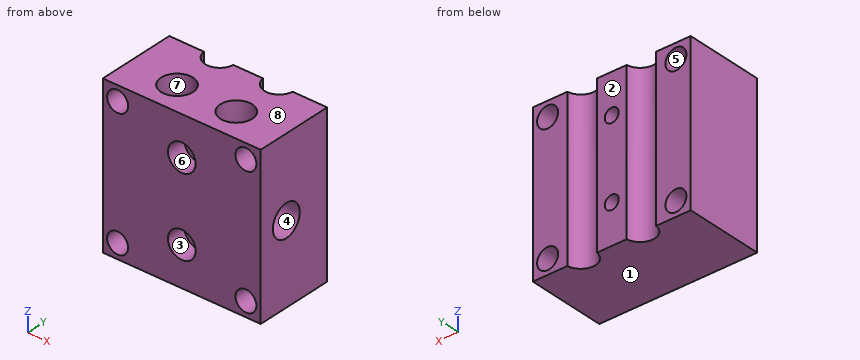
from build123d import *

# Parameters (mm, degrees)
SKETCH1_W                         = 50.8
SKETCH1_H                         = 50.8
BOSS_EXTRUDE1_DEPTH               = 25.4
SKETCH2_R                         = 4.7625
CUT_EXTRUDE1_DEPTH                = 63.217039467
F_1_4_CLEARANCE_HOLE1_D           = 6.7564
F_8_CLEARANCE_HOLE1_D             = 4.4958
SKETCH9_R                         = 4.445
CUT_EXTRUDE3_DEPTH                = 6.35
F_1_8_NPT_TAPPED_HOLE1_AT_2_COUNT = 2
F_1_8_NPT_TAPPED_HOLE1_AT_2_PITCH = 19.05


with BuildPart() as part:
    # Sketch1 → Boss-Extrude1 (new body)
    with BuildSketch(Plane(origin=(0, 0, 0), x_dir=(1, 0, 0), z_dir=(0, 1, 0))):
        Rectangle(SKETCH1_W, SKETCH1_H)
    extrude(amount=BOSS_EXTRUDE1_DEPTH)

    # Sketch2 → Cut-Extrude1 (cut, through all)
    with BuildSketch(Plane.XY.offset(25.4)):
        with Locations((-9.525, 25.908)):
            Circle(SKETCH2_R)
        with Locations((9.525, 25.908)):
            Circle(SKETCH2_R)
    extrude(amount=-CUT_EXTRUDE1_DEPTH, mode=Mode.SUBTRACT)

    # 1/4 Clearance Hole1 (through all)
    with Locations(Plane(origin=(0, 25.4, 0), x_dir=(1, 0, 0), z_dir=(0, 1, 0))):
        with Locations((-20.6375, 20.6375), (-20.6375, -20.6375), (20.6375, -20.6375), (20.6375, 20.6375)):
            Hole(F_1_4_CLEARANCE_HOLE1_D / 2)

    # #8 Clearance Hole1 (through all)
    with Locations(Plane(origin=(0, 25.4, 0), x_dir=(1, 0, 0), z_dir=(0, 1, 0))):
        with Locations((0, 12.7), (0, -12.7)):
            Hole(F_8_CLEARANCE_HOLE1_D / 2)

    # Sketch9 → Cut-Extrude3 (cut)
    with BuildSketch(Plane.XZ):
        with Locations(Location((0, 12.7, 0), (0, 0, 270))):
            Circle(SKETCH9_R)
        with Locations(Location((0, -12.7, 0), (0, 0, 270))):
            Circle(SKETCH9_R)
    extrude(amount=-CUT_EXTRUDE3_DEPTH, mode=Mode.SUBTRACT)

    # Sketch10 → 1/8 NPT Tapped Hole1 (revolve, cut)
    with BuildSketch(Plane(origin=(-9.525, 9.525, 25.4), x_dir=(0, -1, 0), z_dir=(1, 0, 0))):
        Polygon((0, 0), (0, 46.983468714), (4.2164, 44.45), (4.2164, 6.858), (4.936181096, 6.858), (5.1415188, 0), align=None)
    f_1_8_npt_tapped_hole1 = revolve(axis=Axis((-9.525, 9.525, 31.75), (0, 0, -1)), mode=Mode.SUBTRACT)

    # 1/8 NPT Tapped Hole1 at 2: 1/8 NPT Tapped Hole1 ×2
    with Locations(*[(i * F_1_8_NPT_TAPPED_HOLE1_AT_2_PITCH, 0, 0) for i in range(1, F_1_8_NPT_TAPPED_HOLE1_AT_2_COUNT)]):
        add(f_1_8_npt_tapped_hole1, mode=Mode.SUBTRACT)

    # Sketch14 → 1/8 NPT Tapped Hole3 (revolve, cut)
    with BuildSketch(Plane(origin=(25.4, 9.77926984, 0), x_dir=(0, 0, -1), z_dir=(0, 1, 0))):
        Polygon((0, 0), (0, 46.983468714), (4.2164, 44.45), (4.2164, 6.858), (4.936181096, 6.858), (5.1415188, 0), align=None)
    revolve(axis=Axis((31.75, 9.77926984, 0), (-1, 0, 0)), mode=Mode.SUBTRACT)


solid = part.part
Could you check a few things on this model? Use its own coordinates, in mm. Face numbers are marked on the shaded views. A direction names the side the tool comes from. Give positions to 0.01 mm unless a question says otherwise; leave off trailing zeros. Order: outer loops, then holes, each group sorted by start corner. A loop starts at its lowest first (then second) coordinate and runs counter-clockwise, first axis right, second up. Notation, with made-up numbers: (86, -3.75) -> (98, -3.75) arc R27 ccw to (98, 16.25) -> close; hole circle Ø11 at (55.5, 41.25). An arc over 180 degrees is marked (long way). Return JSON: item names as keys, results as strings.
1. For pin 1 Ø5 at (x, z) = (0, -12.7) entering from +Y; pin 2 Ø4 at (x, z) = (20.64, -20.64) entering from +Y; pin 3 Ø2.5 at (x, z) = (1, 14.5) entering from -Y, each with a flat end and sliding along its axis, tell me the tip position at first contact or that it passes through.
Answer list:
{"pin 1": "stops at y = 25.4", "pin 2": "passes through", "pin 3": "stops at y = 6.35"}
2. On a 3-axis mill with a long thin cutter (end or side, diameter ignored), from which of +Z, -Z, +X, -X, +Y, -Y can I reach the whole of each face in a straight line? I mean the marked faces 4, 5, 6, 7 and 8. Say none if no direction works.
Answer list:
{"face 4": "+X", "face 5": "+Y, -Y", "face 6": "-Y", "face 7": "+Z", "face 8": "+Z, +X, -X, +Y, -Y"}
3. Imagine slicing it at D-D on z = -6. List the corners of the cut face in (x, y) for me (1 decimal), then the cut area to 3 significant figures.
Answer list:
{"outline": "(-25.4, 0) -> (25.4, 0) -> (25.4, 25.4) -> (14.3, 25.4) arc R4.8 cw to (4.8, 25.4) -> (-4.8, 25.4) arc R4.8 cw to (-14.3, 25.4) -> (-25.4, 25.4) -> close; hole circle Ø8.4 at (-9.5, 9.5); hole circle Ø8.4 at (9.5, 9.5)", "area": "1,120 mm2"}
4. Thinking about a two-plate mould opening in Z: for the marked faces 1, 2 and 3, which applies, pulls with the +Z half, pulls with the -Z half, needs draft (parallel to the pull), parting line crosses it, or undercut?
Answer list:
{"face 1": "pulls with the -Z half", "face 2": "needs draft", "face 3": "undercut"}
5. Imagine slicing it at A-A on z = 12.7. Give the number of separate pieces and of enclosed holes in the cut face, then the cut area to 3 significant figures.
Answer list:
{"separate pieces": "2", "enclosed holes": "2", "area": "975 mm2"}
6. I need wall thicknesses on line 1 (Y direction, x = 9.5, z = -16.5); line 2 (X direction, y = 21, z = -22.5); line 3 (Z direction, x = -1, y = 9.75). Which ranges of each line are inside material? Lowest first, please. Write a range as from..to.
Answer list:
{"line 1": "y = 0..5.31, 13.74..21.15", "line 2": "x = -25.4..-23.46, -17.82..17.82, 23.46..25.4", "line 3": "z = -25.4..-14.71, -10.69..-4.22, 4.22..10.69, 14.71..25.4"}
7. Imagine slicing it at B-B on x = 0. List the corners of the cut face in (y, z) for me (3 decimals), then the cut area to 3 significant figures.
Answer list:
{"outline": "(0, -25.4) -> (25.4, -25.4) -> (25.4, -14.948) -> (6.35, -14.948) -> (6.35, -17.145) -> (0, -17.145) -> close; (0, -8.255) -> (6.35, -8.255) -> (6.35, -10.452) -> (25.4, -10.452) -> (25.4, 10.452) -> (6.35, 10.452) -> (6.35, 8.255) -> (0, 8.255) -> close; (0, 17.145) -> (6.35, 17.145) -> (6.35, 14.948) -> (25.4, 14.948) -> (25.4, 25.4) -> (0, 25.4) -> close; hole circle Ø8.433 at (9.779, 0)", "area": "950 mm2"}
8. Imagine slicing it at C-C on y = 17.75. List the corners of the cut face in (x, z) for me.
Answer list:
{"outline": "(-25.4, -25.4) -> (25.4, -25.4) -> (25.4, 25.4) -> (-25.4, 25.4) -> close; hole circle Ø6.76 at (-20.64, -20.64); hole circle Ø6.76 at (-20.64, 20.64); hole circle Ø4.5 at (0, -12.7); hole circle Ø4.5 at (0, 12.7); hole circle Ø6.76 at (20.64, -20.64); hole circle Ø6.76 at (20.64, 20.64)"}
